from build123d import *

# Parameters (mm, degrees)
SKETCH1_W           = 2.92
SKETCH1_H           = 2.92
SKETCH1_W_2         = 5.92
BOSS_EXTRUDE1_DEPTH = 3


with BuildPart() as part:
    # Sketch1 → Boss-Extrude1 (new body)
    with BuildSketch(Plane(origin=(0, 0, 0), x_dir=(1, 0, 0), z_dir=(0, 1, 0))):
        with BuildLine():
            Line((-37.489699571, 19.876646482), (-37.489699571, 9.876646482))
            Line((-37.489699571, 9.876646482), (-34.489699571, 9.876646482))
            Line((-34.489699571, 9.876646482), (-34.489699571, 11.876646482))
            ThreePointArc((-34.489699571, 11.876646482), (-34.289699571, 12.876646482), (-34.489699571, 13.876646482))
            Line((-34.489699571, 13.876646482), (-34.489699571, 15.876646482))
            Line((-34.489699571, 15.876646482), (-31.489699571, 15.876646482))
            Line((-31.489699571, 15.876646482), (-31.489699571, 13.876646482))
            ThreePointArc((-31.489699571, 13.876646482), (-31.689699571, 12.876646482), (-31.489699571, 11.876646482))
            Line((-31.489699571, 11.876646482), (-31.489699571, -1.123353518))
            Line((-31.489699571, -1.123353518), (-34.489699571, -1.123353518))
            Line((-34.489699571, -1.123353518), (-34.489699571, -12.123353518))
            Line((-34.489699571, -12.123353518), (-37.489699571, -12.123353518))
            Line((-37.489699571, -12.123353518), (-37.489699571, -22.123353518))
            Line((-37.489699571, -22.123353518), (-34.489699571, -22.123353518))
            Line((-34.489699571, -22.123353518), (-34.489699571, -20.123353518))
            ThreePointArc((-34.489699571, -20.123353518), (-34.289699571, -19.123353518), (-34.489699571, -18.123353518))
            Line((-34.489699571, -18.123353518), (-34.489699571, -16.123353518))
            Line((-34.489699571, -16.123353518), (-31.489699571, -16.123353518))
            Line((-31.489699571, -16.123353518), (-31.489699571, -18.123353518))
            ThreePointArc((-31.489699571, -18.123353518), (-31.689699571, -19.123353518), (-31.489699571, -20.123353518))
            Line((-31.489699571, -20.123353518), (-31.489699571, -25.123353518))
            Line((-31.489699571, -25.123353518), (-23.439699571, -25.123353518))
            Line((-23.439699571, -25.123353518), (-23.439699571, -22.123353518))
            Line((-23.439699571, -22.123353518), (-13.439699571, -22.123353518))
            Line((-13.439699571, -22.123353518), (-13.439699571, -25.123353518))
            Line((-13.439699571, -25.123353518), (-3.439699571, -25.123353518))
            Line((-3.439699571, -25.123353518), (-3.439699571, -22.123353518))
            Line((-3.439699571, -22.123353518), (6.560300429, -22.123353518))
            Line((6.560300429, -22.123353518), (6.560300429, -25.123353518))
            Line((6.560300429, -25.123353518), (16.560300429, -25.123353518))
            Line((16.560300429, -25.123353518), (16.560300429, -22.123353518))
            Line((16.560300429, -22.123353518), (26.560300429, -22.123353518))
            Line((26.560300429, -22.123353518), (26.560300429, -25.123353518))
            Line((26.560300429, -25.123353518), (34.610300429, -25.123353518))
            Line((34.610300429, -25.123353518), (34.610300429, -20.123353518))
            ThreePointArc((34.610300429, -20.123353518), (34.810300429, -19.123353518), (34.610300429, -18.123353518))
            Line((34.610300429, -18.123353518), (34.610300429, -16.123353518))
            Line((34.610300429, -16.123353518), (37.610300429, -16.123353518))
            Line((37.610300429, -16.123353518), (37.610300429, -18.123353518))
            ThreePointArc((37.610300429, -18.123353518), (37.410300429, -19.123353518), (37.610300429, -20.123353518))
            Line((37.610300429, -20.123353518), (37.610300429, -22.123353518))
            Line((37.610300429, -22.123353518), (40.610300429, -22.123353518))
            Line((40.610300429, -22.123353518), (40.610300429, -12.123353518))
            Line((40.610300429, -12.123353518), (37.610300429, -12.123353518))
            Line((37.610300429, -12.123353518), (37.610300429, -1.123353518))
            Line((37.610300429, -1.123353518), (34.610300429, -1.123353518))
            Line((34.610300429, -1.123353518), (34.610300429, 11.876646482))
            ThreePointArc((34.610300429, 11.876646482), (34.810300429, 12.876646482), (34.610300429, 13.876646482))
            Line((34.610300429, 13.876646482), (34.610300429, 15.876646482))
            Line((34.610300429, 15.876646482), (37.610300429, 15.876646482))
            Line((37.610300429, 15.876646482), (37.610300429, 13.876646482))
            ThreePointArc((37.610300429, 13.876646482), (37.410300429, 12.876646482), (37.610300429, 11.876646482))
            Line((37.610300429, 11.876646482), (37.610300429, 9.876646482))
            Line((37.610300429, 9.876646482), (40.610300429, 9.876646482))
            Line((40.610300429, 9.876646482), (40.610300429, 19.876646482))
            Line((40.610300429, 19.876646482), (-37.489699571, 19.876646482))
        make_face()
        with Locations((1.560300429, 16.416646482)):
            Rectangle(SKETCH1_W, SKETCH1_H, mode=Mode.SUBTRACT)
        with Locations((12.870300429, -14.263353518)):
            Rectangle(SKETCH1_W_2, SKETCH1_H, mode=Mode.SUBTRACT)
        with Locations((21.150300429, 10.416646482)):
            Rectangle(SKETCH1_W, SKETCH1_H, mode=Mode.SUBTRACT)
        with Locations((-18.029699571, 10.416646482)):
            Rectangle(SKETCH1_W, SKETCH1_H, mode=Mode.SUBTRACT)
        with Locations((-17.409699571, -14.263353518)):
            Rectangle(SKETCH1_W, SKETCH1_H, mode=Mode.SUBTRACT)
    extrude(amount=BOSS_EXTRUDE1_DEPTH)


solid = part.part
Can you work these out from the model? Positions are in its coordinate system, mm. A direction names the side the tool comes from. Give positions to 0.01 mm unless a question says otherwise; leave off trailing zeros. Order: outer loops, then holes, each group sorted by start corner. A loop starts at its lowest first (then second) coordinate and runs counter-clockwise, first axis right, second up. Notation, with made-up numbers: M 30.5,-20.75 L 63.5,-20.75 A29 cw 63.5,6.25 Z; hole C -27,3.25 d8. An arc over 180 degrees is marked long. Use a Markdown table: item, result. Add a question column.
Item 1: For faces 1 (the flat face through (-19, 1, 22.123)), 2 (the flat face through (3.02, 1, -16)), 3 (the flat face through (36, 1, 1.123)), which set-ups out of +Z, -Z, +X, -X, +Y, -Y let a thin tool reach every point of the face, with its end or its side?
Item 2: If I drill on L1, parallel to X at y = 0.25, z = -13; L2, parallel to X at y = 1.5, z = -14; L3, parallel to X at y = 1.1, z = -16.5, over which ranges is the centre line in solid material (lowest first)? Write a range as [from, to].
Item 3: Will this pin go through, and if not, where does the flat tip stop? pin 1 (0.9 mm diameter, centred on x = -33.5, y = 1.5, fed in from +Z).
Item 4: Suppose I cut it at C-C (z = -3). List the corners of the cut face in (x, y) for me.
Item 5: Suppose I cut it at B-B (y = 2.4). Count the separate pieces of the cut face and the enclosed holes in it, then the cut area to 3 significant figures.
Item 6: Suppose I cut it at A-A (z = 19). List the corners of the cut face in (x, y) for me, then the cut area to 3 significant figures.
Item 7: Suppose I cut it at D-D (x = 4). List the corners of the cut face in (y, z) for me, then the cut area to 3 significant figures.
Item 8: We'd pull the mould along X, two halves only. Please class faces 4 (the flat face through (9.91, 1, 14)), 5 (the flat face through (1, 3, 2)): +X half, -X half, draft (parallel to the pull), parting line (faces both ways), or undercut.
Answer sheet:
| question | item | result |
|---|---|---|
| 1 | face 1 | +Z, +Y, -Y |
| 1 | face 2 | +Y, -Y |
| 1 | face 3 | +X, +Y, -Y |
| 2 | L1 | x = [-37.49, -34.29], [-31.69, 34.81], [37.41, 40.61] |
| 2 | L2 | x = [-37.49, -34.49], [-31.49, 34.61], [37.61, 40.61] |
| 2 | L3 | x = [-37.49, 0.1], [3.02, 40.61] |
| 3 | pin 1 | stops at z = 16.12 |
| 4 | outline | M -31.49,0 L 34.61,0 L 34.61,3 L -31.49,3 Z |
| 5 | separate pieces | 1 |
| 5 | enclosed holes | 5 |
| 5 | area | 3,070 mm² |
| 6 | outline | M -37.49,0 L -34.29,0 L -34.29,3 L -37.49,3 Z; M -31.69,0 L 34.81,0 L 34.81,3 L -31.69,3 Z; M 37.41,0 L 40.61,0 L 40.61,3 L 37.41,3 Z |
| 6 | area | 219 mm² |
| 7 | outline | M 0,-19.88 L 3,-19.88 L 3,22.12 L 0,22.12 Z |
| 7 | area | 126 mm² |
| 8 | face 4 | undercut |
| 8 | face 5 | draft |
